For this review, take the finished solid that the model builds, in its own axes (mm). Round coordinates to 2 decimals unless told otherwise and drop trailing zeros. Answer in a Markdown table with one row per item. Add a question column.
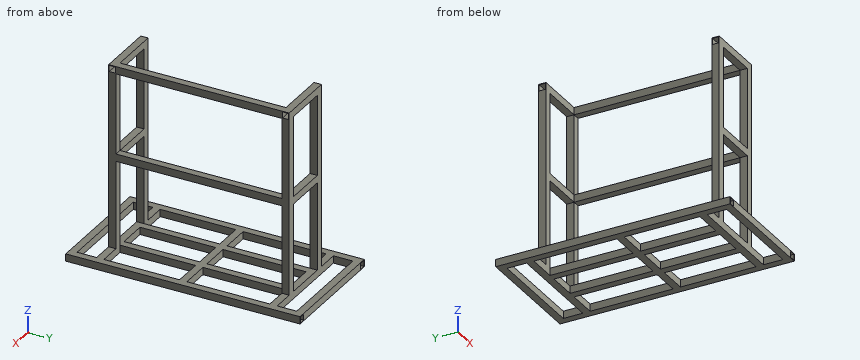
```python
from build123d import *

# Parameters (mm, degrees)
F0_W      = 38.1
F0_H      = 38.1
F0_W_2    = 31.75
F0_H_2    = 31.75
F1_DEPTH  = 1219.2
F2_W      = 38.1
F2_H      = 38.1
F2_W_2    = 31.75
F2_H_2    = 31.75
F3_DEPTH  = 533.4
F4_W      = 38.1
F4_H      = 38.1
F4_W_2    = 31.75
F4_H_2    = 31.75
F5_DEPTH  = 1219.2
F6_W      = 38.1
F6_H      = 38.1
F6_W_2    = 31.75
F6_H_2    = 31.75
F7_DEPTH  = 533.4
F8_W      = 38.1
F8_H      = 38.1
F8_W_2    = 31.75
F8_H_2    = 31.75
F9_DEPTH  = 863.6
F10_W     = 38.1
F10_H     = 38.1
F10_W_2   = 31.75
F10_H_2   = 31.75
F11_DEPTH = 914.4
F12_W     = 38.1
F12_H     = 38.1
F12_W_2   = 31.75
F12_H_2   = 31.75
F13_DEPTH = 304.8
F14_W     = 38.1
F14_H     = 38.1
F14_W_2   = 31.75
F14_H_2   = 31.75
F15_DEPTH = 863.6
F16_W     = 38.1
F16_H     = 38.1
F16_W_2   = 31.75
F16_H_2   = 31.75
F17_DEPTH = 254


with BuildPart() as f1:
    # F0 (on Front) → F1 (new body)
    with BuildSketch(Plane.XZ):
        with Locations((19.05, 19.05)):
            Rectangle(F0_W, F0_H)
        with Locations((19.05, 19.05)):
            Rectangle(F0_W_2, F0_H_2, mode=Mode.SUBTRACT)
    extrude(amount=F1_DEPTH)

    # F2 (on face) → F3 (join)
    with BuildSketch(Plane.YZ.offset(38.1)):
        with Locations((-1200.15, 19.05)):
            Rectangle(F2_W, F2_H)
        with Locations((-1200.15, 19.05)):
            Rectangle(F2_W_2, F2_H_2, mode=Mode.SUBTRACT)
        with Locations((-19.05, 19.05)):
            Rectangle(F2_W, F2_H)
        with Locations((-19.05, 19.05)):
            Rectangle(F2_W_2, F2_H_2, mode=Mode.SUBTRACT)
    extrude(amount=F3_DEPTH)

    # F4 (on face) → F5 (join)
    with BuildSketch(Plane(origin=(0, 0, 0), x_dir=(-1, 0, 0), z_dir=(0, 1, 0))):
        with Locations((-590.55, 19.05)):
            Rectangle(F4_W, F4_H)
        with Locations((-590.55, 19.05)):
            Rectangle(F4_W_2, F4_H_2, mode=Mode.SUBTRACT)
    extrude(amount=-F5_DEPTH)

    # F6 (on face) → F7 (join)
    with BuildSketch(Plane.YZ.offset(38.1)):
        with Locations((-1060.45, 19.05)):
            Rectangle(F6_W, F6_H)
        with Locations((-1060.45, 19.05)):
            Rectangle(F6_W_2, F6_H_2, mode=Mode.SUBTRACT)
        with Locations((-158.75, 19.05)):
            Rectangle(F6_W, F6_H)
        with Locations((-158.75, 19.05)):
            Rectangle(F6_W_2, F6_H_2, mode=Mode.SUBTRACT)
        with Locations((-628.65, 19.05)):
            Rectangle(F6_W, F6_H)
        with Locations((-628.65, 19.05)):
            Rectangle(F6_W_2, F6_H_2, mode=Mode.SUBTRACT)
    extrude(amount=F7_DEPTH)

    # F8 (on face) → F9 (join)
    with BuildSketch(Plane.XZ.offset(177.8)):
        with Locations((209.55, 19.05)):
            Rectangle(F8_W, F8_H)
        with Locations((209.55, 19.05)):
            Rectangle(F8_W_2, F8_H_2, mode=Mode.SUBTRACT)
        with Locations((400.05, 19.05)):
            Rectangle(F8_W, F8_H)
        with Locations((400.05, 19.05)):
            Rectangle(F8_W_2, F8_H_2, mode=Mode.SUBTRACT)
    extrude(amount=F9_DEPTH)

    # F10 (on face) → F11 (join)
    with BuildSketch(Plane.XY.offset(38.1)):
        with Locations((438.15, -158.75)):
            Rectangle(F10_W, F10_H)
        with Locations((438.15, -158.75)):
            Rectangle(F10_W_2, F10_H_2, mode=Mode.SUBTRACT)
        with Locations((171.45, -158.75)):
            Rectangle(F10_W, F10_H)
        with Locations((171.45, -158.75)):
            Rectangle(F10_W_2, F10_H_2, mode=Mode.SUBTRACT)
        with Locations((438.15, -1060.45)):
            Rectangle(F10_W, F10_H)
        with Locations((438.15, -1060.45)):
            Rectangle(F10_W_2, F10_H_2, mode=Mode.SUBTRACT)
        with Locations((171.45, -1060.45)):
            Rectangle(F10_W, F10_H)
        with Locations((171.45, -1060.45)):
            Rectangle(F10_W_2, F10_H_2, mode=Mode.SUBTRACT)
    extrude(amount=F11_DEPTH)

    # F12 (on face) → F13 (join)
    with BuildSketch(Plane(origin=(152.4, 0, 0), x_dir=(0, -1, 0), z_dir=(-1, 0, 0))):
        with Locations((1060.45, 971.55)):
            Rectangle(F12_W, F12_H)
        with Locations((1060.45, 971.55)):
            Rectangle(F12_W_2, F12_H_2, mode=Mode.SUBTRACT)
        with Locations((158.75, 971.55)):
            Rectangle(F12_W, F12_H)
        with Locations((158.75, 971.55)):
            Rectangle(F12_W_2, F12_H_2, mode=Mode.SUBTRACT)
    extrude(amount=-F13_DEPTH)

    # F14 (on face) → F15 (join)
    with BuildSketch(Plane.XZ.offset(177.8)):
        with Locations((438.15, 971.55)):
            Rectangle(F14_W, F14_H)
        with Locations((438.15, 971.55)):
            Rectangle(F14_W_2, F14_H_2, mode=Mode.SUBTRACT)
        with Locations((438.15, 514.35)):
            Rectangle(F14_W, F14_H)
        with Locations((438.15, 514.35)):
            Rectangle(F14_W_2, F14_H_2, mode=Mode.SUBTRACT)
    extrude(amount=F15_DEPTH)

    # F16 (on face) → F17 (join)
    with BuildSketch(Plane(origin=(419.1, 0, 0), x_dir=(0, -1, 0), z_dir=(-1, 0, 0))):
        with Locations((158.75, 514.35)):
            Rectangle(F16_W, F16_H)
        with Locations((158.75, 514.35)):
            Rectangle(F16_W_2, F16_H_2, mode=Mode.SUBTRACT)
        with Locations((1060.45, 514.35)):
            Rectangle(F16_W, F16_H)
        with Locations((1060.45, 514.35)):
            Rectangle(F16_W_2, F16_H_2, mode=Mode.SUBTRACT)
    extrude(amount=F17_DEPTH)


solid = f1.part
```
1. We need section A-A (z = 180.5). Count the separate pieces of the cut face and the enclosed holes in it, plus the area to 3 significant figures.
2. For L1, parallel to Y at x = 444, z = 319.5 (3 decimals); L2, parallel to X at y = -159, z = 127.5 (3 decimals); L3, parallel to Y at x = 189.5, z = 431, list the stretches that pass through material, from the lowest coordinate up. Write a range as [from, to].
3. Clearance check with flat-ended pins moving along their axes: pin 1 Ø5 at (y, z) = (-961.5, 512.5) entering from -X; pin 2 Ø1.5 at (x, z) = (431, 583.5) entering from -Y; pin 3 Ø9.5 at (x, z) = (174.5, 496.5) entering from +Y. State where each tip first meets the part, or that it passes through.
Response:
| question | item | result |
|---|---|---|
| 1 | separate pieces | 4 |
| 1 | enclosed holes | 4 |
| 1 | area | 1,770 mm2 |
| 2 | L1 | [-1079.5, -1076.325], [-1044.575, -1041.4], [-177.8, -174.625], [-142.875, -139.7] |
| 2 | L2 | [152.4, 155.575], [187.325, 190.5], [419.1, 422.275], [454.025, 457.2] |
| 2 | L3 | [-1079.5, -1041.4], [-177.8, -139.7] |
| 3 | pin 1 | x = 419.1 |
| 3 | pin 2 | y = -1079.5 |
| 3 | pin 3 | y = -139.7 |
